Here's how the part is built. I have some questions about the finished solid (model axes, mm). Round coordinates to 2 decimals unless told otherwise and drop trailing zeros. Write each loop counter-clockwise with the first axis right and the second up, starting at its lowest first coordinate (ties: lowest second). Pieces come first, ordered by that corner, then holes. Notation, with made-up numbers: (-9, 66) -> (29, 66) arc R22 ccw to (29, 94) -> close; hole circle Ø6 at (-36, -5.75). An arc over 180 degrees is marked (long way). Answer as CSV lines item,"result".
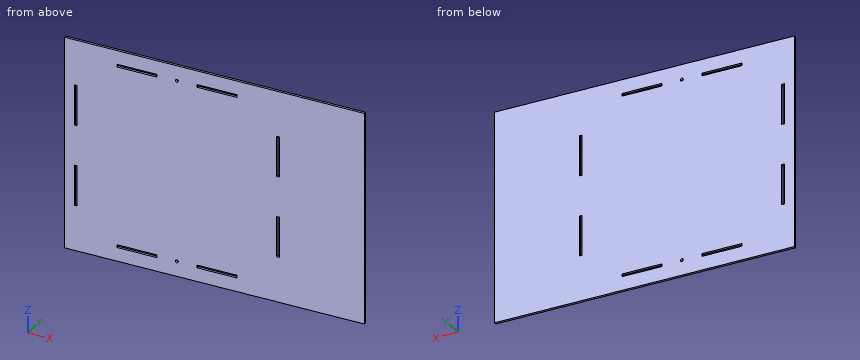
```python
from build123d import *

# Parameters (mm, degrees)
SKETCH1_W           = 300
SKETCH1_H           = 210
BOSS_EXTRUDE1_DEPTH = 2.5
SKETCH4_W           = 2.7
SKETCH4_H           = 40
SKETCH4_W_2         = 40
SKETCH4_H_2         = 2.7
SKETCH4_R           = 1.5
CUT_EXTRUDE1_DEPTH  = 2.5


with BuildPart() as part:
    # Sketch1 → Boss-Extrude1 (new body)
    with BuildSketch(Plane(origin=(0, 0, 0), x_dir=(1, 0, 0), z_dir=(0, 1, 0))):
        Rectangle(SKETCH1_W, SKETCH1_H)
    extrude(amount=BOSS_EXTRUDE1_DEPTH)

    # Sketch4 → Cut-Extrude1 (cut)
    with BuildSketch(Plane(origin=(0, 2.5, 0), x_dir=(1, 0, 0), z_dir=(0, 1, 0))):
        with Locations((-138.65, 40)):
            Rectangle(SKETCH4_W, SKETCH4_H)
        with Locations((-138.65, -40)):
            Rectangle(SKETCH4_W, SKETCH4_H)
        with Locations((-77.5, -90)):
            Rectangle(SKETCH4_W_2, SKETCH4_H_2)
        with Locations(Location((-37.5, -90, 0), (0, 0, 270))):
            Circle(SKETCH4_R)
        with Locations((2.5, -90)):
            Rectangle(SKETCH4_W_2, SKETCH4_H_2)
        with Locations((63.65, 40)):
            Rectangle(SKETCH4_W, SKETCH4_H)
        with Locations((63.65, -40)):
            Rectangle(SKETCH4_W, SKETCH4_H)
        with Locations(Location((-37.5, 90, 0), (0, 0, 270))):
            Circle(SKETCH4_R)
        with Locations((-77.5, 90)):
            Rectangle(SKETCH4_W_2, SKETCH4_H_2)
        with Locations((2.5, 90)):
            Rectangle(SKETCH4_W_2, SKETCH4_H_2)
    extrude(amount=-CUT_EXTRUDE1_DEPTH, mode=Mode.SUBTRACT)


solid = part.part
```
1. Suppose I cut it at A-A on z = 47.5. Please give me the cut outline in (x, y).
Numbers:
outline,"(-150, 0) -> (-140, 0) -> (-140, 2.5) -> (-150, 2.5) -> close; (-137.3, 0) -> (62.3, 0) -> (62.3, 2.5) -> (-137.3, 2.5) -> close; (65, 0) -> (150, 0) -> (150, 2.5) -> (65, 2.5) -> close"
2. If I drill on line 1 (Z direction, x = 62.5, y = 0.95); line 2 (X direction, y = 0.85, z = 90); line 3 (Z direction, x = -62, y = 0.3), over which ranges is the centre line in solid material (lowest first)?
Numbers:
line 1,"z = -105 to -60, -20 to 20, 60 to 105"
line 2,"x = -150 to -97.5, -57.5 to -39, -36 to -17.5, 22.5 to 150"
line 3,"z = -105 to -91.35, -88.65 to 88.65, 91.35 to 105"
3. Suppose I cut it at B-B on x = -12.5. Please give me the cut outline in (y, z).
Numbers:
outline,"(0, -105) -> (2.5, -105) -> (2.5, -91.35) -> (0, -91.35) -> close; (0, -88.65) -> (2.5, -88.65) -> (2.5, 88.65) -> (0, 88.65) -> close; (0, 91.35) -> (2.5, 91.35) -> (2.5, 105) -> (0, 105) -> close"
